from build123d import *

# Parameters (mm, degrees)
F0_R     = 100
F0_W     = 7
F0_H     = 60
F0_H_2   = 2
F0_W_2   = 2
F0_H_3   = 56
F1_DEPTH = 2
F2_DEPTH = 25


# Not quite as in the source:
# - a feature names something its author has since deleted; it is built from what else it names


with BuildPart() as f1:
    # F0 (on Top) → F1 (new body)
    with BuildSketch(Plane.XY):
        Circle(F0_R)
        with Locations((-83.5, 0)):
            Rectangle(F0_W, F0_H, mode=Mode.SUBTRACT)
        Polygon((-58.5, 30), (-56.5, 30), (-49.5, 30), (-49.5, 28), (-56.5, 28), (-56.5, -28), (-49.5, -28), (-49.5, -30), (-56.5, -30), (-58.5, -30), (-65.5, -30), (-65.5, -28), (-58.5, -28), (-58.5, 28), (-65.5, 28), (-65.5, 30), align=None, mode=Mode.SUBTRACT)
        with Locations((83.5, 0)):
            Rectangle(F0_W, F0_H, mode=Mode.SUBTRACT)
        with Locations((-62, -29)):
            Rectangle(F0_W, F0_H_2)
        with Locations((-57.5, -29)):
            Rectangle(F0_W_2, F0_H_2)
        with Locations((-53, -29)):
            Rectangle(F0_W, F0_H_2)
        with Locations((-57.5, 0)):
            Rectangle(F0_W_2, F0_H_3)
        with Locations((-62, 29)):
            Rectangle(F0_W, F0_H_2)
        with Locations((-57.5, 29)):
            Rectangle(F0_W_2, F0_H_2)
        with Locations((-53, 29)):
            Rectangle(F0_W, F0_H_2)
    extrude(amount=F1_DEPTH)

    # F0 (on Top) → F2 (join)
    with BuildSketch(Plane.XY):
        with Locations((-62, 29)):
            Rectangle(F0_W, F0_H_2)
        with Locations((-57.5, 29)):
            Rectangle(F0_W_2, F0_H_2)
        with Locations((-53, 29)):
            Rectangle(F0_W, F0_H_2)
        with Locations((-57.5, 0)):
            Rectangle(F0_W_2, F0_H_3)
        with Locations((-62, -29)):
            Rectangle(F0_W, F0_H_2)
        with Locations((-57.5, -29)):
            Rectangle(F0_W_2, F0_H_2)
        with Locations((-53, -29)):
            Rectangle(F0_W, F0_H_2)
    extrude(amount=F2_DEPTH)


solid = f1.part
CAD build for the part. Positions are in the model's coordinates, mm. A direction names the side the tool comes from. Round coordinates to 2 decimals unless told otherwise and drop trailing zeros. Order: outer loops, then holes, each group sorted by start corner. A loop starts at its lowest first (then second) coordinate and runs counter-clockwise, first axis right, second up. Notation, with made-up numbers: M -7,2 L 51,2 A20 cw 51,24 Z; hole C -14.75,-9.5 d7. An arc over 180 degrees is marked long. Use one line per item in the form item = value.
Q1. Saw through at C-C on x = 0. Give the cut face in (y, z).
Recorded:
outline = M -100,0 L 100,0 L 100,2 L -100,2 Z
Q2. Probe L1, parallel to Z at x = -66, y = 60; L2, parallel to Y at x = -81, z = 1.75; L3, parallel to X at y = -13, z = 3. List the from-to ranges inside material, lowest first.
Recorded:
L1 = 0 to 2
L2 = -58.64 to -30, 30 to 58.64
L3 = -58.5 to -56.5
Q3. Saw through at D-D on y = -73. Give the cut face in (x, z), then the cut area to 3 significant figures.
Recorded:
outline = M -68.34,0 L 68.34,0 L 68.34,2 L -68.34,2 Z
area = 273 mm^2
Q4. Saw through at B-B on z = 17.75. Give the cut face in (x, y), then the cut area to 3 significant figures.
Recorded:
outline = M -65.5,-30 L -49.5,-30 L -49.5,-28 L -56.5,-28 L -56.5,28 L -49.5,28 L -49.5,30 L -65.5,30 L -65.5,28 L -58.5,28 L -58.5,-28 L -65.5,-28 Z
area = 176 mm^2
Q5. Two-plate mould, pull along Y, no slides. Class faces 1 (the cylindrical face through (95.38, 30.04, 0.99)), 2 (the flat face through (-57, 30, 13)), 3 (the flat face through (-62, -28, 13)): +Y half, -Y half, draft (parallel to the pull), parting line (faces both ways), or undercut.
Recorded:
face_1 = parting line
face_2 = +Y half
face_3 = undercut
Q6. Flat gauge pins, fed straight in: P1, Ø6, axis at y = -14, z = 20, coming from the +X side; P2, Ø5.5, axis at x = -53.5, z = 15, coming from the -Y side; P3, Ø12, axis at x = -3, y = -17, coming from the +Z side. Where does each tip first touch, or does it go through?
Recorded:
P1 = -56.5
P2 = -30
P3 = 2
Q7. Which spindle directions (+Z, -Z, +X, -X, +Y, -Y) get a long thin tool onto all of the face, cutting with end or side? Do faces 4 (the flat face through (-56.5, 0, 13)), 5 (the flat face through (-58.5, 0, 13)), 6 (the flat face through (-58, 0, 25)), 7 (the flat face through (-58, -30, 13)). Say none if no direction does.
Recorded:
face_4 = +Z, +X
face_5 = +Z, -X
face_6 = +Z, +X, -X, +Y, -Y
face_7 = +Z, +X, -X, -Y
Q8. Saw through at A-A on y = 0. Give the cut face in (x, z).
Recorded:
outline = M -100,0 L -87,0 L -87,2 L -100,2 Z; M -80,0 L 80,0 L 80,2 L -56.5,2 L -56.5,25 L -58.5,25 L -58.5,2 L -80,2 Z; M 87,0 L 100,0 L 100,2 L 87,2 Z
